Part print with two shaded views. Sizes in mm from the minimum x, y, z corner. Round coordinates to 2 decimals unless told otherwise and drop trailing zeros. Write each loop counter-clockwise with the first axis right and the second up, starting at its lowest first coordinate (ties: lowest second). Pieces come first, ordered by that corner, then holes. Notation, with made-up numbers: (-12, 46) -> (14, 46) arc R17 cw to (14, 66) -> close; hole circle Ø8 at (49.5, 61). An arc over 180 degrees is marked (long way). Put each result on its own line as item: value. Start each with the question number.
1. Pull direction Y, two halves, no side cores. Call the marked faces 1, 2 and 3: pulls with the +Y half, pulls with the -Y half, needs draft (parallel to the pull), parting line crosses it, or undercut.
2. Saw through at D-D on y = 30.5. List the corners of the cut face in (x, z) (1 decimal).
3. Drill centre lines: line 1 (Y direction, x = 7, z = 19); line 2 (Z direction, x = 2.75, y = 14.5) (1 decimal); line 3 (Y direction, x = 4, z = 17). Where is each one in solid material? Low to high. Write a range as from..to.
4. Saw through at A-A on x = 7.25. List the corners of the cut face in (y, z).
5. Saw through at C-C on y = 16. List the corners of the cut face in (x, z) (1 decimal), and give its area (3 significant figures).
6. Saw through at B-B on z = 24. List the corners of the cut face in (x, y), and give its area (3 significant figures).
7. Flat gauge pin, fed straight in: P1, Ø5, axis at y = 12, z = 15, coming from the +X side. Where does the tip first touch, or does it go through?
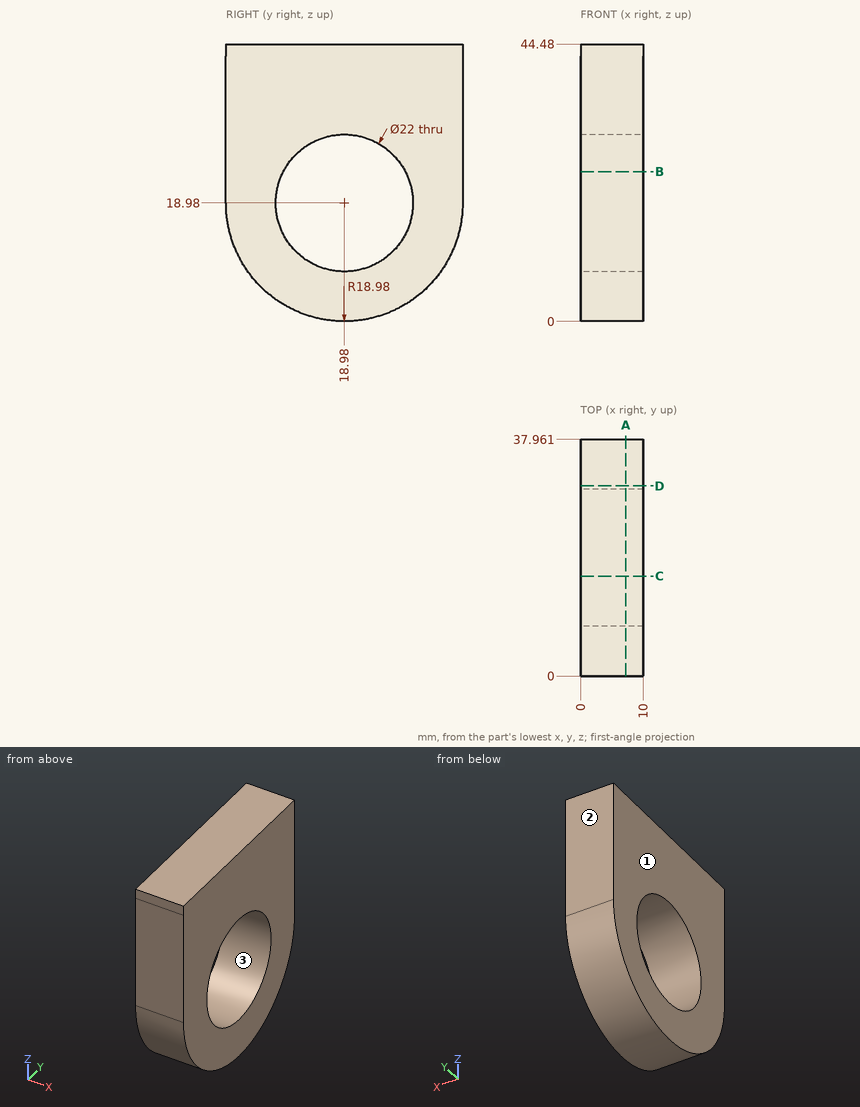
Return value:
1. face 1: needs draft
1. face 2: pulls with the +Y half
1. face 3: undercut
2. outline: (0, 3.9) -> (10, 3.9) -> (10, 44.5) -> (0, 44.5) -> close
3. line 1: y = 0..7.98, 29.98..37.96
3. line 2: z = 0.5..8.9, 29..44.5
3. line 3: y = 0.1..8.16, 29.8..37.86
4. outline: (0, 18.98) arc R18.98 ccw to (37.96, 18.98) -> (37.96, 44.48) -> (0, 44.48) -> close; hole circle Ø22 at (18.98, 18.98)
5. outline: (0, 0.2) -> (10, 0.2) -> (10, 8.4) -> (0, 8.4) -> close; (0, 29.6) -> (10, 29.6) -> (10, 44.5) -> (0, 44.5) -> close
5. area: 231 mm^2
6. outline: (0, 0) -> (10, 0) -> (10, 9.19) -> (0, 9.19) -> close; (0, 28.77) -> (10, 28.77) -> (10, 37.96) -> (0, 37.96) -> close
6. area: 184 mm^2
7. P1: passes through
